Autodesk Inventor part; units mm, degrees
ref_plane "YZ Plane" through (0, 0, 0) normal (1, 0, 0) x (0, 1, 0)
ref_plane "XZ Plane" through (0, 0, 0) normal (0, 1, 0) x (-1, 0, 0)
ref_plane "XY Plane" through (0, 0, 0) normal (0, 0, 1) x (1, 0, 0)
sketch "Szkic1" plane through (0, 0, 0) normal (0, 1, 0) x (-1, 0, 0)
  line L0 (11.7026, 13.5166) -> (-11.1274, 13.5166)
  line L1 (-11.1274, 13.5166) -> (-11.1274, -17.4543)
  line L2 (-11.1274, -17.4543) -> (11.7026, -17.4543)
  line L3 (11.7026, -17.4543) -> (11.7026, 13.5166)
  point P0 (0, 0)
extrude "Wyciągnięcie proste1" add sketch "Szkic1" along normal blind 2
sketch "Szkic2" plane through (0, 2, 0) normal (0, 1, 0) x (1, 0, 0)
  line L0 (11.1274, 17.4543) -> (-11.7026, 17.4543)
  line L1 (-7.7876, 7.4543) -> (7.2124, 7.4543)
  line L2 (7.2124, 7.4543) -> (7.2124, 17.4543)
  line L3 (7.2124, 17.4543) -> (-7.7876, 17.4543)
  line L4 (-7.7876, 17.4543) -> (-7.7876, 7.4543)
  point P0 (0, 0)
  point P1 (-0.2876, 7.4543)
  point P2 (-0.2876, 17.4543)
  dimension "d2" = 15
  dimension "d3" = 10
extrude "Wyciągnięcie proste2" add sketch "Szkic2" along normal blind 15
fillet "Zaokrąglenie1" radius 5 2 edges at (-0.2876, 17, -7.4543) (-0.2876, 17, -17.4543)
sketch "Szkic3" plane through (7.2124, 2, -7.4543) normal (1, 0, 0) x (0, 0, -1)
  arc A0 (10, 10) -> (0, 10) centre (5, 10) ccw
  line L0 (0, 0) -> (0, 10)
  line L1 (10, 0) -> (0, 0)
  line L2 (10, 0) -> (10, 10)
  circle A1 centre (5, 10) radius 1.5
  point P0 (-7.4543, -2)
  dimension "d7" = 3
extrude "Wyciągnięcie proste3" cut sketch "Szkic3" against normal blind 15 contours A1
properties part number "uchwyt"
The listing builds one solid part. Answer for the finished solid, in the listing's coordinates (mm). A direction names the side the tool comes from. Coordinates: 2 decimals unless noted, no trailing zeros. Order: outer loops, then holes, each group sorted by start corner. A loop starts at its lowest first (then second) coordinate and runs counter-clockwise, first axis right, second up. Notation, with made-up numbers: M -13,55.5 L 23,55.5 A15 ccw 23,62.5 Z; hole C -2.5,-38.5 d9. An arc over 180 degrees is marked long. Use CSV: the item, a comma, the result in double quotes.
Q1. Determine the mould class of faces 1 (the flat face through (0, 0, -2)), 2 (the cylindrical face through (-0.183, 12.066, -10.956)), 3 (the cylindrical face through (-0.183, 15.574, -8.958)), 4 (the flat face through (-11.703, 1, -2)) for opening direction Y: pulls with the +Y half, pulls with the -Y half, needs draft (parallel to the pull), parting line crosses it, or undercut.
Here are the results:
face 1,"pulls with the -Y half"
face 2,"undercut"
face 3,"pulls with the +Y half"
face 4,"needs draft"
Q2. Section D-D (y = 9) is taken. Determine the outline of the cut face in (x, z), then the cut area to 3 significant figures.
Here are the results:
outline,"M -7.79,-17.45 L 7.21,-17.45 L 7.21,-7.45 L -7.79,-7.45 Z"
area,"150 mm2"
Q3. Section C-C (z = -4) is taken. Determine the outline of the cut face in (x, y), then the cut area to 3 significant figures.
Here are the results:
outline,"M -11.7,0 L 11.13,0 L 11.13,2 L -11.7,2 Z"
area,"45.7 mm2"
Q4. A tool of negligible diameter and unlimited length cuts with its end or side. For faces 5 (the flat face through (-7.788, 9, -13)), 6 (the flat face through (0, 7, -7.454)), 7 (the flat face through (7.212, 9, -12)), 8 (the flat face through (0, 6, -17.454)), from which of +Z, -Z, +X, -X, +Y, -Y can it reach the whole face along a straight path? Write none if from no direction.
Here are the results:
face 5,"+Z, -Z, -X, +Y"
face 6,"+Z, +X, -X, +Y"
face 7,"+Z, -Z, +X, +Y"
face 8,"-Z, +X, -X, +Y, -Y"
Q5. Section B-B (y = 11) is taken. Determine the outline of the cut face in (x, z), then the cut area to 3 significant figures.
Here are the results:
outline,"M -7.79,-17.45 L 7.21,-17.45 L 7.21,-13.57 L -7.79,-13.57 Z; M -7.79,-11.34 L 7.21,-11.34 L 7.21,-7.45 L -7.79,-7.45 Z"
area,"116 mm2"
Q6. Straight lines are drawn through the part: L1, parallel to Z at x = -5.5, y = 10; L2, parallel to X at y = 6, z = -12; L3, parallel to Y at x = 7.25, z = -4.5. For each, find the intervals that lie inside material, in ascending order.
Here are the results:
L1,"-17.45 to -7.45"
L2,"-7.79 to 7.21"
L3,"0 to 2"
Q7. Given pin 1 Ø11.5 at (x, z) = (-4, 0.5) entering from +Y; pin 2 Ø1 at (x, y) = (-7.5, 10.5) entering from +Z; pin 3 Ø5 at (y, z) = (7.5, -14) entering from +X, each flat-ended and moving along its own axis, determine where each tip first touches the part or whether it passes through.
Here are the results:
pin 1,"y = 2"
pin 2,"z = -7.45"
pin 3,"x = 7.21"
